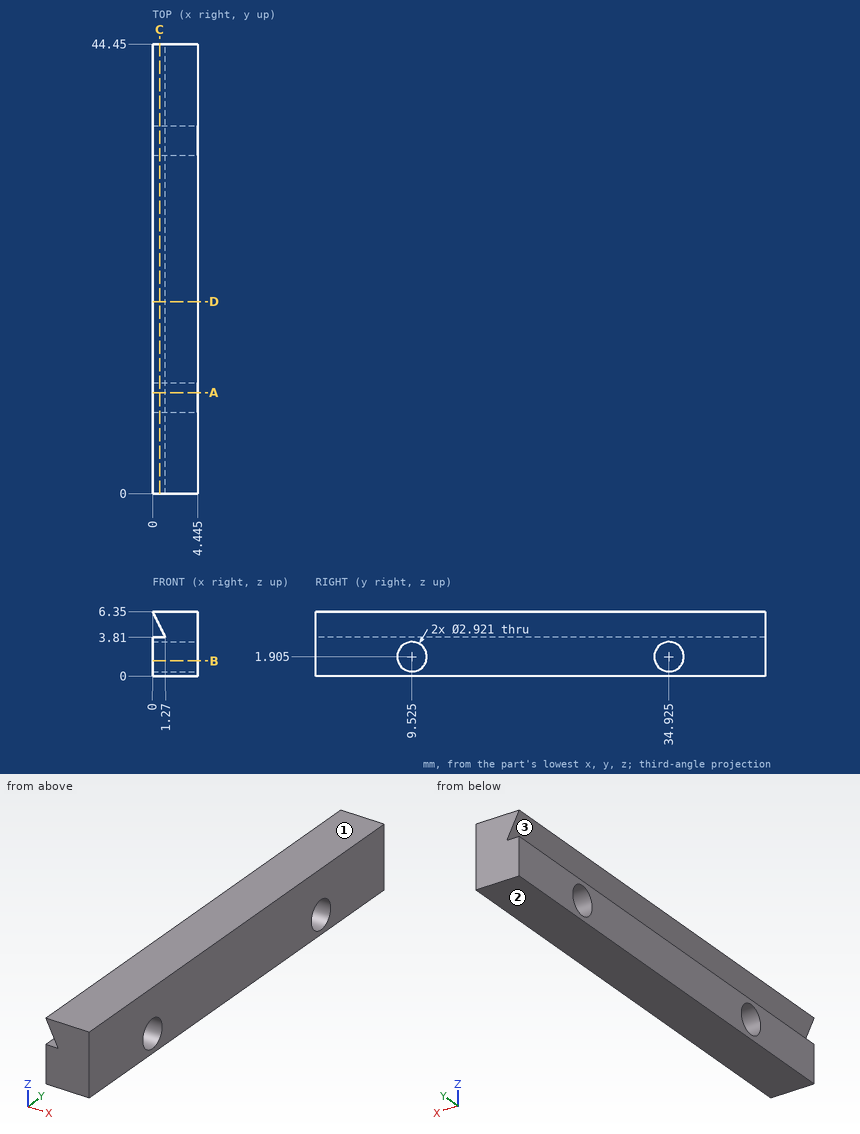
Here's the drawing with two shaded views (mm, measured from the low corner). I have some questions. Coordinates: 2 decimals unless noted, no trailing zeros. Loops run counter-clockwise (first coordinate to the right, second up) from the corner with the lowest first, then second, coordinate; pieces in that order, holes last. Notation, with made-up numbers: (89.25, 6) - (119.25, 6) arc R20 cw to (119.25, 42) - close; hole circle Ø1 at (37, -13.5). An arc over 180 degrees is marked (long way). Answer as CSV lines item,"result". Start each with the question number.
1) Suppose I cut it at C-C (x = 0.7). Count the separate pieces of the cut face and the enclosed holes in it, plus the area to 3 significant figures.
2) Suppose I cut it at B-B (z = 1.5). Please give me the cut outline in (x, y) (3 decimals).
3) Suppose I cut it at A-A (y = 10). Please give me the cut outline in (x, z) (3 decimals), plus the area to 3 significant figures.
4) Thinking about a two-plate mould opening in Z: for the marked faces 1, 2 and 3, which applies, pulls with the +Z half, pulls with the -Z half, needs draft (parallel to the pull), parting line crosses it, or undercut?
5) I need wall thicknesses on line 1 (Y direction, x = 1.6, z = 1.75); line 2 (Z direction, x = 1, y = 8.5); line 3 (Y direction, x = 2.7, z = 1.5). Which ranges of each line are inside material? Lowest first, please. Write a range as from..to.
6) Suppose I cut it at D-D (y = 19). Please give me the cut outline in (x, z) (3 decimals).
7) For pin 1 (2.5 mm diameter, centred on y = 9.525, z = 1.905, fed in from +X); pin 2 (3 mm diameter, centred on y = 18, z = 4.5, fed in from -X), each with a flat end and sliding along its axis, tell me the tip position at first contact or that it passes through.
Check result:
1,separate pieces,"2"
1,enclosed holes,"2"
1,area,"218 mm²"
2,outline,"(0, 0) - (4.445, 0) - (4.445, 8.122) - (0, 8.122) - close; (0, 10.928) - (4.445, 10.928) - (4.445, 33.522) - (0, 33.522) - close; (0, 36.328) - (4.445, 36.328) - (4.445, 44.45) - (0, 44.45) - close"
3,outline,"(0, 0) - (4.445, 0) - (4.445, 0.524) - (0, 0.524) - close; (0, 3.286) - (4.445, 3.286) - (4.445, 6.35) - (0, 6.35) - (1.27, 3.81) - (0, 3.81) - close"
3,area,"14.3 mm²"
4,face 1,"pulls with the +Z half"
4,face 2,"pulls with the -Z half"
4,face 3,"undercut"
5,line 1,"y = 0..8.07, 10.98..33.47, 36.38..44.45"
5,line 2,"z = 0..0.86, 2.95..3.81, 4.35..6.35"
5,line 3,"y = 0..8.12, 10.93..33.52, 36.33..44.45"
6,outline,"(0, 0) - (4.445, 0) - (4.445, 6.35) - (0, 6.35) - (1.27, 3.81) - (0, 3.81) - close"
7,pin 1,"passes through"
7,pin 2,"stops at x = 0"
